The model under review builds one solid part; all positions refer to its coordinate system, in mm. Coordinates: 2 decimals unless noted, no trailing zeros. Write each loop counter-clockwise with the first axis right and the second up, starting at its lowest first coordinate (ties: lowest second). Pieces come first, ordered by that corner, then holes. Notation, with made-up numbers: (69, 84) - (127, 84) arc R29 cw to (127, 121) - close; hole circle Ø7 at (47.25, 46). An arc over 180 degrees is marked (long way). Put each result on its own line as item: value.
Solid Edge part; units mm, degrees
sketch "Sketch1" plane through (0, 0, 0) normal (0, 0, 1) x (1, 0, 0)
  line L0 (-69.5, -25) -> (69.5, -25)
  line L1 (69.5, -25) -> (69.5, 25)
  line L2 (69.5, 25) -> (-69.5, 25)
  line L3 (-69.5, 25) -> (-69.5, -25)
  dimension "D1" = 69.5
  dimension "D2" = 69.5
extrude "Protrusion1" add sketch "Sketch1" along normal mid plane 4
sketch "Sketch2" plane through (0, 0, 2) normal (0, 0, 1) x (1, 0, 0)
  line L0 (-39.495, -25) -> (-29.505, -25)
  line L1 (-29.505, -25) -> (-29.505, -21)
  line L2 (-29.505, -21) -> (-39.495, -21)
  line L3 (-39.495, -21) -> (-39.495, -25)
  line L4 (-19.495, -25) -> (-9.505, -25)
  line L5 (-9.505, -25) -> (-9.505, -21)
  line L6 (-9.505, -21) -> (-19.495, -21)
  line L7 (-19.495, -21) -> (-19.495, -25)
  line L8 (0.505, -25) -> (10.495, -25)
  line L9 (10.495, -25) -> (10.495, -21)
  line L10 (10.495, -21) -> (0.505, -21)
  line L11 (0.505, -21) -> (0.505, -25)
  line L12 (20.505, -25) -> (30.495, -25)
  line L13 (30.495, -25) -> (30.495, -21)
  line L14 (30.495, -21) -> (20.505, -21)
  line L15 (20.505, -21) -> (20.505, -25)
  line L16 (40.505, -25) -> (50.495, -25)
  line L17 (50.495, -25) -> (50.495, -21)
  line L18 (50.495, -21) -> (40.505, -21)
  line L19 (40.505, -21) -> (40.505, -25)
  line L20 (60.505, -25) -> (70.495, -25)
  line L21 (70.495, -25) -> (70.495, -21)
  line L22 (70.495, -21) -> (60.505, -21)
  line L23 (60.505, -21) -> (60.505, -25)
  line L24 (-59.495, -25) -> (-49.505, -25)
  line L25 (-49.505, -25) -> (-49.505, -21)
  line L26 (-49.505, -21) -> (-59.495, -21)
  line L27 (-59.495, -21) -> (-59.495, -25)
  dimension "D1" = 49.505
  dimension "D2" = 29.505
  dimension "D3" = 50.495
  dimension "D4" = 30.495
  dimension "D5" = 9.505
  dimension "D6" = 10.495
  dimension "D7" = 59.495
  dimension "D8" = 39.495
  dimension "D9" = 19.495
  dimension "D10" = 0.505
  dimension "D11" = 20.505
  dimension "D12" = 40.505
  dimension "D13" = 60.505
  dimension "D14" = 70.495
extrude "Extrusionsausschnitt_1" cut sketch "Sketch2" against normal blind 200
mirror "Mirror1" about plane through (0, 0, 0) normal (0, -1, 0) of "Extrusionsausschnitt_1"
properties material "Holz, Kiefer"
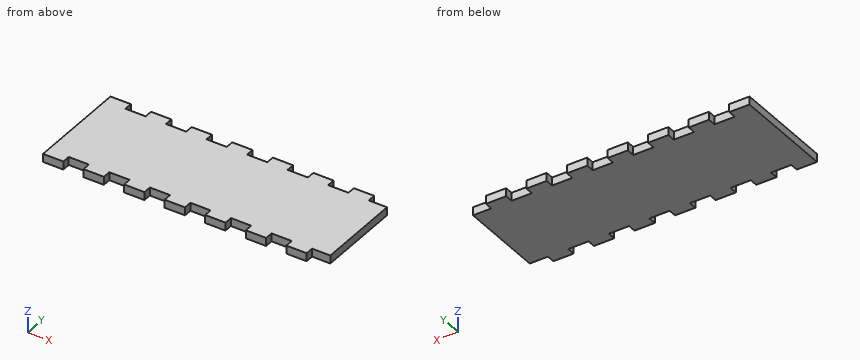
1. To check wall thickness, follow probe 1 along Y at (x, z) = (-50, 0.5). State the ranges of the line that lie inside material, in increasing order.
Determined:
probe 1: y = -21 to 21
2. Consider section A-A on x = -57.5. State the section outline as (y, z) points, plus the area to 3 significant figures.
Determined:
outline: (-21, -2) - (21, -2) - (21, 2) - (-21, 2) - close
area: 168 mm^2
3. For pin 1 Ø1.2 at (y, z) = (-23, -1) entering from +X (3 decimals); pin 2 Ø1.2 at (x, z) = (-53.5, 1) entering from +Y; pin 3 Ø2 at (x, z) = (-52, 0) entering from -Y, all flat-tipped, find the tip position at first contact; note any pin that passes through.
Determined:
pin 1: stops at x = 60.505
pin 2: stops at y = 21
pin 3: stops at y = -21
